Autodesk Inventor part; units mm, degrees
ref_plane "YZ Plane" through (0, 0, 0) normal (1, 0, 0) x (0, 1, 0)
ref_plane "XZ Plane" through (0, 0, 0) normal (0, 1, 0) x (-1, 0, 0)
ref_plane "XY Plane" through (0, 0, 0) normal (0, 0, 1) x (1, 0, 0)
sketch "Sketch1" plane through (0, 0, 0) normal (0, 0, 1) x (1, 0, 0)
  line L0 (0, 0) -> (25.4, 0)
  line L1 (25.4, 0) -> (25.4, 25.4)
  line L2 (25.4, 25.4) -> (0, 25.4)
  line L3 (0, 25.4) -> (0, 0)
  line L4 (3.175, 22.225) -> (22.225, 22.225)
  line L5 (22.225, 22.225) -> (22.225, 3.175)
  line L6 (22.225, 3.175) -> (3.175, 3.175)
  line L7 (3.175, 3.175) -> (3.175, 22.225)
  dimension "d0" = 25.4
  dimension "d1" = 25.4
  dimension "d2" = 3.175
extrude "Extrusion1" add sketch "Sketch1" along normal blind 101.6
sketch "Sketch2" plane through (25.4, 0, 0) normal (1, 0, 0) x (0, 0, -1)
  line L0 (-101.6, 0) -> (-101.6, 25.4)
  line L1 (0, 0) -> (-101.6, 0)
  circle A0 centre (-88.9, 12.7) radius 2.0701
  circle A1 centre (-76.2, 12.7) radius 2.0701
  circle A2 centre (-63.5, 12.7) radius 2.0701
  circle A3 centre (-50.8, 12.7) radius 2.0701
  dimension "d5" = 4.1402
  dimension "d6" = 12.7
  dimension "d7" = 12.7
  dimension "d10" = 12.7
extrude "Extrusion2" cut sketch "Sketch2" against normal blind 101.6
sketch "Sketch3" plane through (0, 25.4, 0) normal (0, 1, 0) x (1, 0, 0)
  line L0 (25.4, 0) -> (0, 0)
  line L1 (25.4, 0) -> (25.4, -101.6)
  circle A0 centre (12.7, -12.7) radius 2.0701
  circle A1 centre (12.7, -38.1) radius 2.0701
  dimension "d17" = 4.1402
  dimension "d18" = 12.7
  dimension "d19" = 12.7
  dimension "d22" = 25.4
extrude "Extrusion3" cut sketch "Sketch3" against normal blind 101.6
properties part number "Clapper Pneumatic Supports (2)"
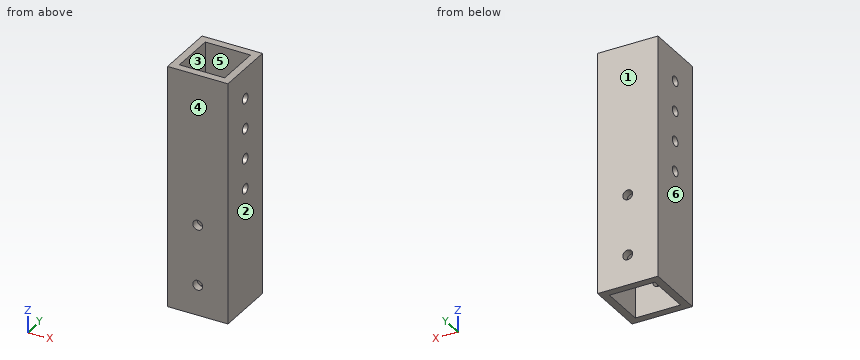
Can you work these out from the model? Positions are in its coordinate system, mm. Face numbers are marked on the shaded views. A direction names the side the tool comes from. Round coordinates to 2 decimals unless told otherwise and drop trailing zeros. Write each loop counter-clockwise with the first axis right and the second up, starting at its lowest first coordinate (ties: lowest second). Pieces come first, ordered by that corner, then holes. Notation, with made-up numbers: (57.25, 67) -> (81.25, 67) arc R14 ccw to (81.25, 80) -> close; hole circle Ø4 at (13, 89.25). An arc over 180 degrees is marked (long way). One line per question, with ' | ' between items. Start each with the question number.
1) Suppose I cut it at B-B on y = 20.75. Write out the boundary of the cut face in (x, z) (3 decimals).
2) If we mould it in two halves opening along Y, with no side actions, what happens to the marked faces 1, 2, 3 and 4? For each: released by +Y, released by -Y, zero draft, split by the parting line, or undercut.
3) Suppose I cut it at A-A on z = 38.1. Write out the boundary of the cut face in (x, y) (3 decimals).
4) Suppose I cut it at D-D on z = 26. Write out the boundary of the cut face in (x, y) (3 decimals).
5) On a 3-axis mill with a long thin cutter (end or side, diameter ignored), from which of +Z, -Z, +X, -X, +Y, -Y can I reach the whole of each face in a straight line? I mean the marked faces 5 and 6. Say none if no direction works.
6) I need wall thicknesses on line 1 (Y direction, x = 7.25, z = 86.5) (3 decimals); line 2 (X direction, y = 1.25, z = 12.7). Which ranges of each line are inside material? Lowest first, please. Write a range as [from, to].
7) I'm going to push a flat-ended pin straight in: P1, Ø12, axis at x = 3.5, z = 23, coming from the -Y side. Where does the tip first touch, or does it pass through?
Return value:
1) outline: (0, 0) -> (3.175, 0) -> (3.175, 101.6) -> (0, 101.6) -> close; (22.225, 0) -> (25.4, 0) -> (25.4, 101.6) -> (22.225, 101.6) -> close
2) face 1: released by +Y | face 2: zero draft | face 3: undercut | face 4: released by -Y
3) outline: (0, 0) -> (10.63, 0) -> (10.63, 3.175) -> (3.175, 3.175) -> (3.175, 22.225) -> (10.63, 22.225) -> (10.63, 25.4) -> (0, 25.4) -> close; (14.77, 0) -> (25.4, 0) -> (25.4, 25.4) -> (14.77, 25.4) -> (14.77, 22.225) -> (22.225, 22.225) -> (22.225, 3.175) -> (14.77, 3.175) -> close
4) outline: (0, 0) -> (25.4, 0) -> (25.4, 25.4) -> (0, 25.4) -> close; hole (3.175, 3.175) -> (22.225, 3.175) -> (22.225, 22.225) -> (3.175, 22.225) -> close
5) face 5: +Z, -Z | face 6: +Z, -Z, -X, +Y, -Y
6) line 1: y = [0, 3.175], [22.225, 25.4] | line 2: x = [0, 10.63], [14.77, 25.4]
7) P1: stops at y = 0
